Check sheet for the drawn part. Datum: minimum x, y, z corner. Units: mm. A direction names the side the tool comes from. Round coordinates to 2 decimals unless told otherwise and drop trailing zeros. Write each loop counter-clockwise with the first axis right and the second up, starting at its lowest first coordinate (ties: lowest second). Pieces come first, ordered by that corner, then holes. Notation, with made-up numbers: (75, 55) - (111, 55) arc R21 cw to (111, 76) - close; hole circle Ø1 at (56, 17). An arc over 180 degrees is marked (long way). Answer as a JSON object with one key per item and string values. Group by question number.
Item 1: Thickness scan on line 1 (X direction, y = 9, z = 6.75); line 2 (X direction, y = 7.75, z = 5.25) (1 decimal); line 3 (Z direction, x = 6, y = 1.75). Record the ranges inside material, lowest first.
Item 2: Set-up check for the marked faces 1 and 2: record each of +Z, -Z, +X, -X, +Y, -Y from which the full face is reachable in a straight line by a thin tool's end or side.
Item 3: Sectioned sample at B-B on y = 5. Record the boundary of the cut face in (x, z).
Item 4: Gauge pin test, flat ends, axial feed: P1, Ø5, axis at y = 9, z = 11, coming from the -X side; P2, Ø3, axis at x = 7, z = 7, coming from the +Y side; P3, Ø1.5, axis at x = 12.5, z = 5, coming from the +Y side; P4, Ø4, axis at x = 11.5, y = 7.5, coming from the -Z side. Record the tip position at first contact, or that the pin passes through.
Item 5: Sectioned sample at A-A on y = 15. Record the boundary of the cut face in (x, z), plus the area to 3 significant figures.
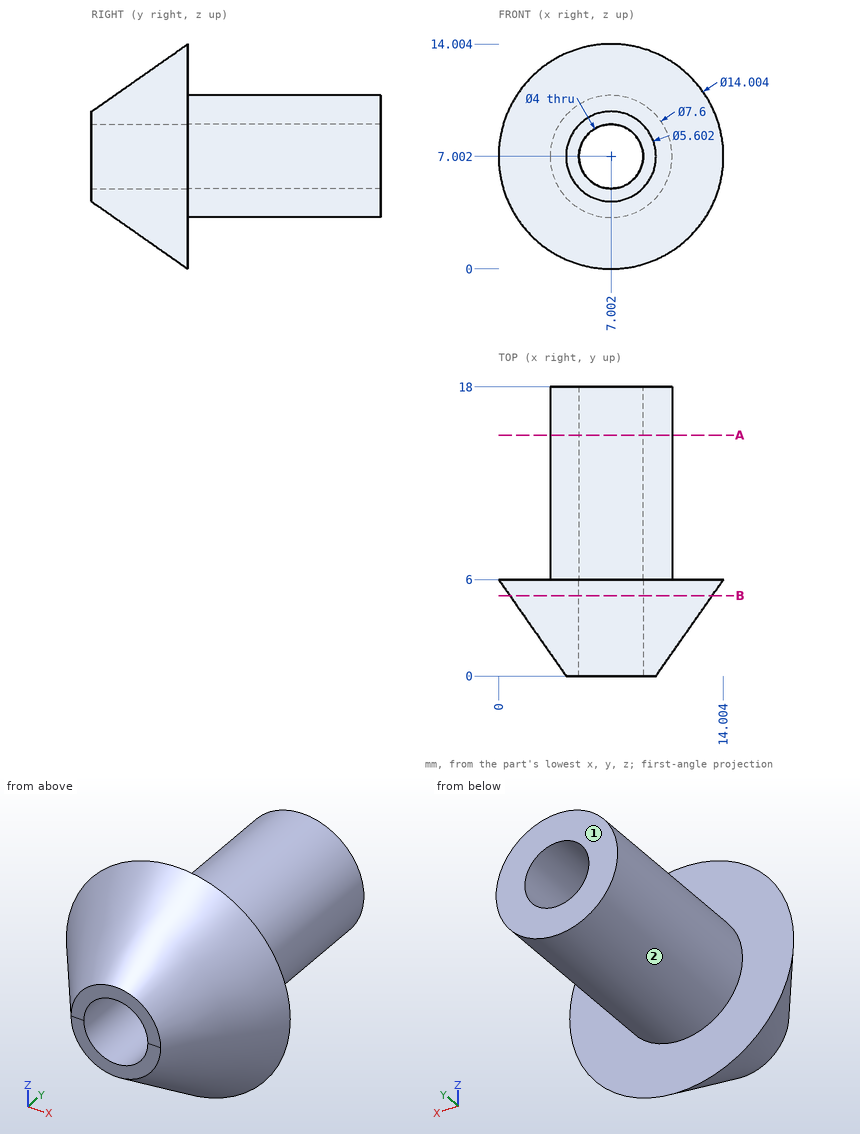
Completed:
{
 "1": {"line 1": "3.21 to 5.02, 8.99 to 10.79", "line 2": "3.6 to 6, 8 to 10.4", "line 3": "3.1 to 5.27, 8.73 to 10.9"},
 "2": {"face 1": "+Z, -Z, +X, -X, +Y", "face 2": "+Y"},
 "3": {"outline": "circle Ø12.6 at (7, 7); hole circle Ø4 at (7, 7)"},
 "4": {"P1": "x = 3.51", "P2": "through", "P3": "y = 6", "P4": "z = 0.76"},
 "5": {"outline": "circle Ø7.6 at (7, 7); hole circle Ø4 at (7, 7)", "area": "32.8 mm²"}
}
